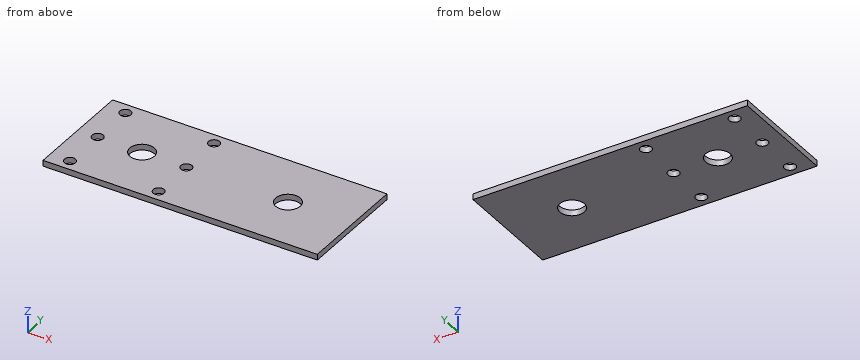
```python
from build123d import *

# Parameters (mm, degrees)
F0_W     = 119.38
F0_H     = 48.26
F0_R     = 5.334
F1_DEPTH = 2.54
F2_DEPTH = 2.54
F3_R     = 2.413
F4_DEPTH = 2.541
F5_R     = 2.413
F6_DEPTH = 2.541


with BuildPart() as f1:
    # F0 (on Top) → F1 (new body)
    with BuildSketch(Plane.XY):
        Rectangle(F0_W, F0_H)
        with Locations((-31.75, 0)):
            Circle(F0_R, mode=Mode.SUBTRACT)
        with Locations((31.75, 0)):
            Circle(F0_R, mode=Mode.SUBTRACT)
    extrude(amount=F1_DEPTH)

    # F0 (on Top) → F2 (join)
    with BuildSketch(Plane.XY):
        Rectangle(F0_W, F0_H)
        with Locations((-31.75, 0)):
            Circle(F0_R, mode=Mode.SUBTRACT)
        with Locations((31.75, 0)):
            Circle(F0_R, mode=Mode.SUBTRACT)
    extrude(amount=F2_DEPTH)

    # F3 (on face) → F4 (cut, through all)
    with BuildSketch(Plane.XY.offset(2.54)):
        with Locations((-51.054, 0)):
            Circle(F3_R)
        with Locations((-51.054, 19.177)):
            Circle(F3_R)
        with Locations((-51.054, -19.177)):
            Circle(F3_R)
    extrude(amount=-F4_DEPTH, mode=Mode.SUBTRACT)

    # F5 (on face) → F6 (cut, through all)
    with BuildSketch(Plane.XY.offset(2.54)):
        with Locations((-12.446, 0)):
            Circle(F5_R)
        with Locations((-12.446, 19.177)):
            Circle(F5_R)
        with Locations((-12.446, -19.177)):
            Circle(F5_R)
    extrude(amount=-F6_DEPTH, mode=Mode.SUBTRACT)


solid = f1.part
```
Here's how the part is built. I have some questions about the finished solid (model axes, mm). Round coordinates to 2 decimals unless told otherwise and drop trailing zeros. Write each loop counter-clockwise with the first axis right and the second up, starting at its lowest first coordinate (ties: lowest second). Pieces come first, ordered by that corner, then holes.
Q1. If we section it at A-A on x = 31.75: Write out the boundary of the cut face in (y, z).
Q2. If we section it at C-C on z = 0.65: Give the number of separate pieces and of enclosed holes in the cut face, plus the area to 3 significant figures.
Q3. If we section it at B-B on y = 0: Write out the boundary of the cut face in (x, z).
Q4. Please list where these lines run through material, in increasing order: probe 1 along X at (y, z) = (17, 2.3); probe 2 along X at (y, z) = (3, 0.6); probe 3 along X at (y, z) = (0.5, 2.05).
Q5. If we section it at D-D on x = -13.5: Write out the boundary of the cut face in (y, z).
Q6. Will this pin go through, and if not, where does the flat tip stop? P1, Ø3, axis at x = -51.054, y = -19.177, coming from the -Z side.
Answer below:
1. outline: (-24.13, 0) - (-5.33, 0) - (-5.33, 2.54) - (-24.13, 2.54) - close; (5.33, 0) - (24.13, 0) - (24.13, 2.54) - (5.33, 2.54) - close
2. separate pieces: 1
2. enclosed holes: 8
2. area: 5,470 mm2
3. outline: (-59.69, 0) - (-53.47, 0) - (-53.47, 2.54) - (-59.69, 2.54) - close; (-48.64, 0) - (-37.08, 0) - (-37.08, 2.54) - (-48.64, 2.54) - close; (-26.42, 0) - (-14.86, 0) - (-14.86, 2.54) - (-26.42, 2.54) - close; (-10.03, 0) - (26.42, 0) - (26.42, 2.54) - (-10.03, 2.54) - close; (37.08, 0) - (59.69, 0) - (59.69, 2.54) - (37.08, 2.54) - close
4. probe 1: x = -59.69 to -52.09, -50.01 to -13.49, -11.41 to 59.69
4. probe 2: x = -59.69 to -36.16, -27.34 to 27.34, 36.16 to 59.69
4. probe 3: x = -59.69 to -53.41, -48.69 to -37.06, -26.44 to -14.81, -10.09 to 26.44, 37.06 to 59.69
5. outline: (-24.13, 0) - (-21.35, 0) - (-21.35, 2.54) - (-24.13, 2.54) - close; (-17.01, 0) - (-2.17, 0) - (-2.17, 2.54) - (-17.01, 2.54) - close; (2.17, 0) - (17.01, 0) - (17.01, 2.54) - (2.17, 2.54) - close; (21.35, 0) - (24.13, 0) - (24.13, 2.54) - (21.35, 2.54) - close
6. P1: passes through
